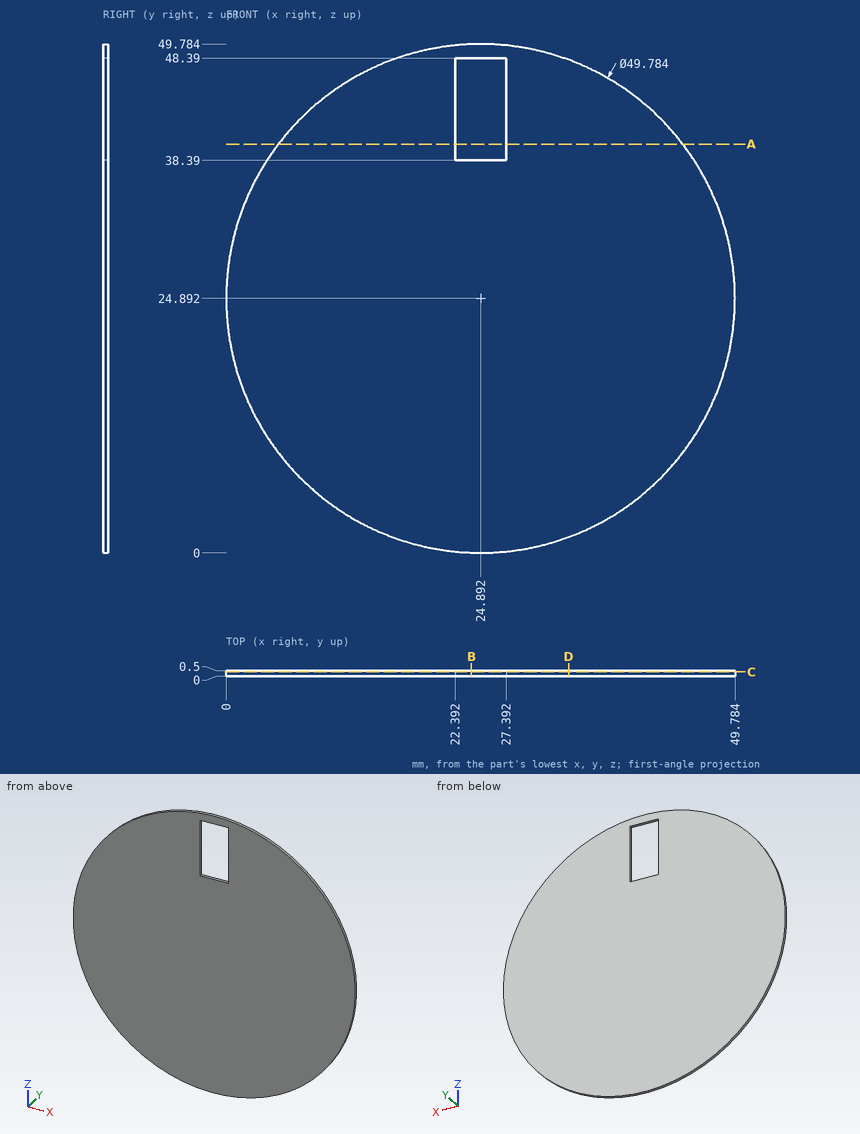
Could you check a few things on this drawing? It's one solid part, dimensions in mm from its lowest x, y, z. Give positions to 0.01 mm unless a question says otherwise; leave off trailing zeros. Order: outer loops, then holes, each group sorted by start corner. A loop starts at its lowest first (then second) coordinate and runs counter-clockwise, first axis right, second up. Notation, with made-up numbers: M 14,-12 L 65,-12 A28 ccw 65,27 Z; hole C 8.25,81 d5. An arc over 180 degrees is marked long. Use one line per item in the form item = value.
Item 1: If we section it at A-A, the plane z = 40: Write out the boundary of the cut face in (x, y) (3 decimals), and give its area (3 significant figures).
Values follow:
outline = M 5.109,0 L 22.392,0 L 22.392,0.5 L 5.109,0.5 Z; M 27.392,0 L 44.675,0 L 44.675,0.5 L 27.392,0.5 Z
area = 17.3 mm^2
Item 2: If we section it at C-C, the plane y = 0.4: Write out the boundary of the cut face in (x, z), and give its area (3 significant figures).
Values follow:
outline = C 24.89,24.89 d49.78; hole M 22.39,38.39 L 27.39,38.39 L 27.39,48.39 L 22.39,48.39 Z
area = 1,900 mm^2
Item 3: If we section it at D-D, the plane x = 33.5: Write out the boundary of the cut face in (y, z).
Values follow:
outline = M 0,1.54 L 0.5,1.54 L 0.5,48.25 L 0,48.25 Z
Item 4: If we section it at B-B, the plane x = 24: Write out the boundary of the cut face in (y, z).
Values follow:
outline = M 0,0.02 L 0.5,0.02 L 0.5,38.39 L 0,38.39 Z; M 0,48.39 L 0.5,48.39 L 0.5,49.77 L 0,49.77 Z
Item 5: If I drill on line 1 along X through (y, z) = (0.4, 42); line 2 along Z through (x, y) = (23, 0.15); line 3 along X through (y, z) = (0.45, 40.5), over which ranges is the centre line in solid material (lowest first)? Write a range as [from, to].
Values follow:
line_1 = [6.81, 22.39], [27.39, 42.97]
line_2 = [0.07, 38.39], [48.39, 49.71]
line_3 = [5.5, 22.39], [27.39, 44.28]
